from build123d import *

# Parameters (mm, degrees)
RING_START                = 3.18
RING_SKETCH_R             = 99
RING_SKETCH_R_2           = 85
RING_SKETCH_R_3           = 1.5
RING_DEPTH                = 6.35
WALL_START                = -91
WALL_SCREW_HOLES_SKETCH_R = 1.65
WALL_SCREW_HOLES_DEPTH    = 9
WALL_SCREW_HOLES_X8_COUNT = 8


with BuildPart() as part:
    # Ring Sketch → Ring (new body)
    with BuildSketch(Plane(origin=(0, 0, 0), x_dir=(0, 0, -1), z_dir=(1, 0, 0)).offset(RING_START)):
        Circle(RING_SKETCH_R)
        Circle(RING_SKETCH_R_2, mode=Mode.SUBTRACT)
        with Locations((0, 92)):
            Circle(RING_SKETCH_R_3, mode=Mode.SUBTRACT)
        with Locations((-92, 0)):
            Circle(RING_SKETCH_R_3, mode=Mode.SUBTRACT)
        with Locations((0, -92)):
            Circle(RING_SKETCH_R_3, mode=Mode.SUBTRACT)
        with Locations((92, 0)):
            Circle(RING_SKETCH_R_3, mode=Mode.SUBTRACT)
    extrude(amount=RING_DEPTH)

    # Wall Screw Holes Sketch → Wall Screw Holes (cut)
    with BuildSketch(Plane(origin=(0, 0, 0), x_dir=(-1, 0, 0), z_dir=(0, -0.9238795325112867, -0.3826834323650897)).offset(WALL_START)):
        with Locations(Location((-6.355, 0, 0), (0, 0, 90))):
            Circle(WALL_SCREW_HOLES_SKETCH_R)
    wall_screw_holes = extrude(amount=-WALL_SCREW_HOLES_DEPTH, mode=Mode.SUBTRACT)

    # Wall Screw Holes x8: Wall Screw Holes ×8 about axis
    wall_screw_holes_x8_axis = Axis((0, 0, 0), (1, 0, 0))
    for i in range(1, WALL_SCREW_HOLES_X8_COUNT):
        add(wall_screw_holes.rotate(wall_screw_holes_x8_axis, i * 360 / WALL_SCREW_HOLES_X8_COUNT), mode=Mode.SUBTRACT)


solid = part.part
For this review, take the finished solid that the model builds, in its own axes (mm). Round coordinates to 2 decimals unless told otherwise and drop trailing zeros. Write each loop counter-clockwise with the first axis right and the second up, starting at its lowest first coordinate (ties: lowest second). Pieces come first, ordered by that corner, then holes. Notation, with made-up numbers: M 62.5,87 L 79.5,87 A20 ccw 79.5,96 Z; hole C 4.5,78.25 d9. An arc over 180 degrees is marked long. Write item = value, one per line. Start each with the question number.
(1) Clearance check with flat-ended pins moving along their axes: pin 1 Ø2.5 at (y, z) = (0, -92) entering from -X; pin 2 Ø1 at (x, z) = (7.5, 20) entering from -Y; pin 3 Ø3.5 at (y, z) = (-92, 0) entering from +X; pin 4 Ø3 at (x, y) = (6, -51.5) entering from -Z. State where each tip first meets the part, or that it passes through.
(2) For line 1 along Y through (x, z) = (7.5, 0); line 2 along Y through (x, z) = (6.75, -36); line 3 along Z through (x, y) = (6.5, -92), list the stretches that pass through material, from the lowest coordinate up.
(3) We need section B-B (z = -5). Give the boundary of the cut face in (x, y).
(4) The part is to be moulded in two halves that separate along X. For faces 1 (the face through (9.53, 74, -44)), 2 (the face through (6.311, -51.721, 67.453)), 3 (the face through (6.43, -87.09, -37.86)), say which applies: +X half, -X half, draft (parallel to the pull), parting line (faces both ways), or undercut.
(5) We need section A-A (y = -8). Give the boundary of the cut face in (x, z), then the cut area to 3 significant figures.
Results found:
q1.pin_1 = through
q1.pin_2 = -97.06
q1.pin_3 = 9.53
q1.pin_4 = -85.45
q2.line_1 = -99 to -93.5, -90.5 to -85, 85 to 90.5, 93.5 to 99
q2.line_2 = -92.22 to -91.1, -83.59 to -77, 77 to 83.59, 91.1 to 92.22
q2.line_3 = -36.33 to -1.5, 1.5 to 36.33
q3.outline = M 3.18,-98.87 L 9.53,-98.87 L 9.53,-84.85 L 3.18,-84.85 Z; M 3.18,84.85 L 9.53,84.85 L 9.53,98.87 L 3.18,98.87 Z
q4.face_1 = +X half
q4.face_2 = draft
q4.face_3 = undercut
q5.outline = M 3.18,-98.68 L 9.53,-98.68 L 9.53,-84.62 L 3.18,-84.62 Z; M 3.18,84.62 L 9.53,84.62 L 9.53,98.68 L 3.18,98.68 Z
q5.area = 178 mm²
